Study the drawing (mm; zero at the part's minimum x, y, z) and answer. A direction names the side the tool comes from. Round coordinates to 2 decimals unless told otherwise and drop trailing zeros. Write each loop counter-clockwise with the first axis right and the second up, starting at its lowest first coordinate (ties: lowest second). Pieces come first, ordered by that corner, then holes.
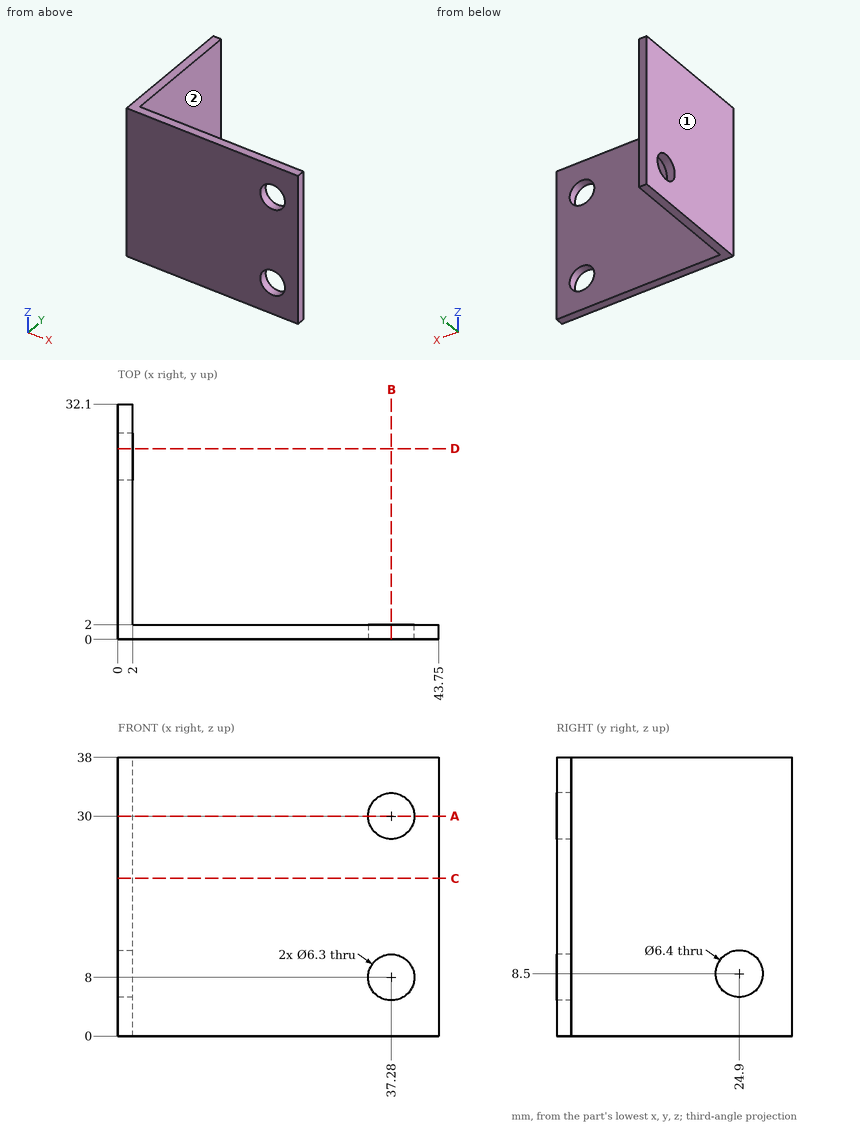
1. A tool of negligible diameter and unlimited length cuts with its end or side. For the marked faces 1 and 2, from which of +Z, -Z, +X, -X, +Y, -Y can it reach the whole face along a straight path? Write none if from no direction.
Geometry says:
face 1: +Z, -Z, -X, +Y, -Y
face 2: +Z, -Z, +X, +Y
2. Given pin 1 (8.5 mm diameter, centred on y = 24.9, z = 8.5, fed in from +X); pin 2 (5 mm diameter, centred on x = 5, y = 11, fed in from +Z); pin 3 (1 mm diameter, centred on x = 20, z = 33.5, fed in from -Y); pin 4 (8 mm diameter, centred on x = 28, z = 26, fed in from +Y), each flat-ended and moving along its own axis, determine where each tip first touches the part or whether it passes through.
Geometry says:
pin 1: stops at x = 2
pin 2: passes through
pin 3: stops at y = 0
pin 4: stops at y = 2
3. Straight lines are drawn through the part: line 1 along Z through (x, y) = (37.28, 0.6); line 2 along X through (y, z) = (1, 30); line 3 along Y through (x, z) = (8.5, 9.5). For each, find the intervals that lie inside material, in ascending order.
Geometry says:
line 1: z = 0 to 4.85, 11.15 to 26.85, 33.15 to 38
line 2: x = 0 to 34.13, 40.43 to 43.75
line 3: y = 0 to 2
4. Section B-B on x = 37.28 is taken. Determine the outline of the cut face in (y, z).
Geometry says:
outline: (0, 0) - (2, 0) - (2, 4.85) - (0, 4.85) - close; (0, 11.15) - (2, 11.15) - (2, 26.85) - (0, 26.85) - close; (0, 33.15) - (2, 33.15) - (2, 38) - (0, 38) - close
5. Section D-D on y = 26 is taken. Determine the outline of the cut face in (x, z) (3 decimals).
Geometry says:
outline: (0, 0) - (2, 0) - (2, 5.495) - (0, 5.495) - close; (0, 11.505) - (2, 11.505) - (2, 38) - (0, 38) - close
6. Section C-C on z = 21.5 is taken. Determine the outline of the cut face in (x, y), plus the area to 3 significant figures.
Geometry says:
outline: (0, 0) - (43.75, 0) - (43.75, 2) - (2, 2) - (2, 32.1) - (0, 32.1) - close
area: 148 mm2
7. Section A-A on z = 30 is taken. Determine the outline of the cut face in (x, y), plus the area to 3 significant figures.
Geometry says:
outline: (0, 0) - (34.13, 0) - (34.13, 2) - (2, 2) - (2, 32.1) - (0, 32.1) - close; (40.43, 0) - (43.75, 0) - (43.75, 2) - (40.43, 2) - close
area: 135 mm2
